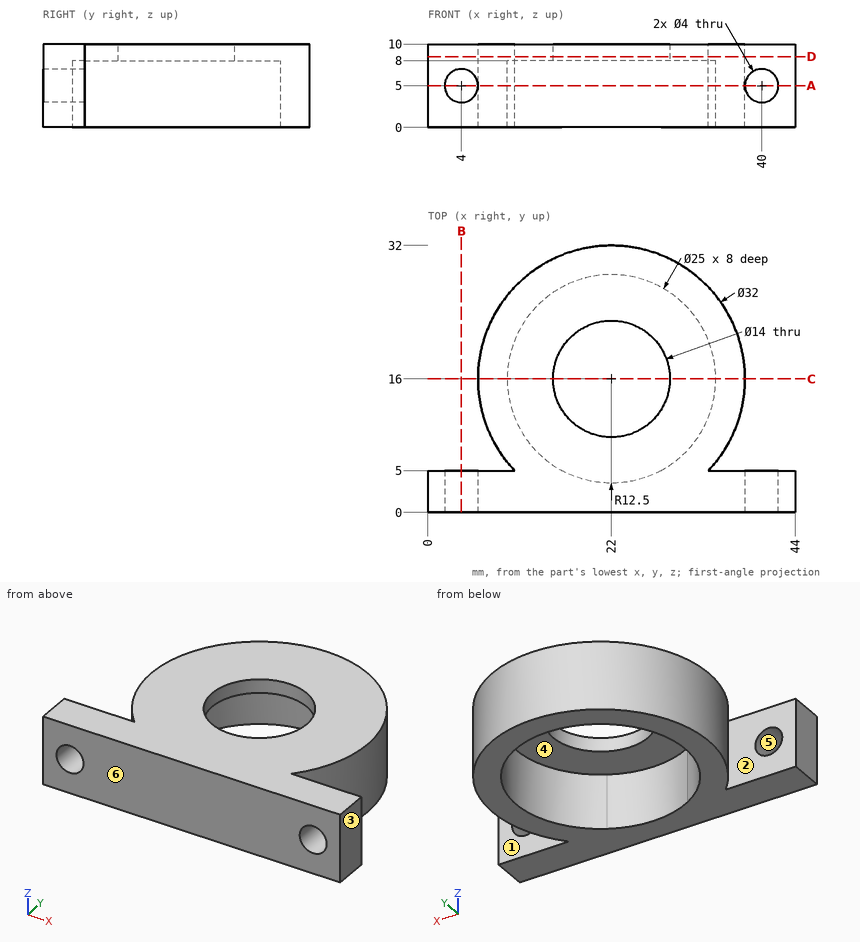
Could you check a few things on this drawing? It's one solid part, dimensions in mm from its lowest x, y, z. A direction names the side the tool comes from. Coordinates: 2 decimals unless noted, no trailing zeros. Write each loop counter-clockwise with the first axis right and the second up, starting at its lowest first coordinate (ties: lowest second). Pieces come first, ordered by that corner, then holes.
Q1. Imagine slicing it at A-A, the plane z = 5. List the corners of the cut face in (x, y) for me, plus the area to 3 significant figures.
Results found:
outline: (0, 0) - (2, 0) - (2, 5) - (0, 5) - close; (6, 0) - (38, 0) - (38, 5) - (33.62, 5) arc R16 ccw (long way) to (10.38, 5) - (6, 5) - close; (42, 0) - (44, 0) - (44, 5) - (42, 5) - close; hole circle Ø25 at (22, 16)
area: 413 mm2
Q2. For P1, Ø3, axis at y = 21, z = 8.5, coming from the +X side; P2, Ø5, axis at x = 37.5, z = 4, coming from the +Y side; P3, Ø6, axis at y = 23.5, z = 4.5, coming from the +X side, each with a flat end and sliding along its axis, tell me the tip position at first contact or that it passes through.
Results found:
P1: stops at x = 37.61
P2: stops at y = 25.33
P3: stops at x = 37.35
Q3. Which directions (+Z, -Z, +X, -X, +Y, -Y) give clear straight access to the entire face, cutting with the end or side of a thin tool? Please do the marked faces 1, 2 and 3.
Results found:
face 1: +Z, -Z, +X
face 2: +Z, -Z, -X
face 3: +Z, -Z, +X, +Y, -Y
Q4. Imagine slicing it at D-D, the plane z = 8.5. List the corners of the cut face in (x, y) for me.
Results found:
outline: (0, 0) - (44, 0) - (44, 5) - (33.62, 5) arc R16 ccw (long way) to (10.38, 5) - (0, 5) - close; hole circle Ø14 at (22, 16)
Q5. If we mould it in two halves opening along Z, with no side actions, what happens to the marked faces 4, 5 and 6? For each: +Z half, -Z half, draft (parallel to the pull), parting line (faces both ways), or undercut.
Results found:
face 4: -Z half
face 5: undercut
face 6: draft
Q6. Imagine slicing it at B-B, the plane x = 4. List the corners of the cut face in (y, z) for me, plus the area to 3 significant figures.
Results found:
outline: (0, 0) - (5, 0) - (5, 3) - (0, 3) - close; (0, 7) - (5, 7) - (5, 10) - (0, 10) - close
area: 30.0 mm2
Q7. Imagine slicing it at C-C, the plane y = 16. List the corners of the cut face in (x, z) for me, plus the area to 3 significant figures.
Results found:
outline: (6, 0) - (9.5, 0) - (9.5, 8) - (15, 8) - (15, 10) - (6, 10) - close; (29, 8) - (34.5, 8) - (34.5, 0) - (38, 0) - (38, 10) - (29, 10) - close
area: 92.0 mm2
Q8. Please list where these lines run through material, in increasing order: L1, parallel to Y at x = 22, z = 9.15; L2, parallel to Y at x = 22, z = 4.25; L3, parallel to X at y = 7.5, z = 5.5.
Results found:
L1: y = 0 to 9, 23 to 32
L2: y = 0 to 3.5, 28.5 to 32
L3: x = 8.44 to 12.83, 31.17 to 35.56
